from build123d import *

# Parameters (mm, degrees)
F_5_0MM_DOWEL_HOLE1_D                     = 5
F_5_0MM_DOWEL_HOLE1_DEPTH                 = 12
F_5_0MM_DOWEL_HOLE1_CSINK_D               = 5.05
F_5_0MM_DOWEL_HOLE1_CSINK_ANGLE           = 90
F_5_0MM_DOWEL_HOLE1_TIP                   = 1.502151548
F_5_0MM_DOWEL_HOLE1_ON_FACE_2_D           = 5
F_5_0MM_DOWEL_HOLE1_ON_FACE_2_DEPTH       = 12
F_5_0MM_DOWEL_HOLE1_ON_FACE_2_CSINK_D     = 5.05
F_5_0MM_DOWEL_HOLE1_ON_FACE_2_CSINK_ANGLE = 90
F_5_0MM_DOWEL_HOLE1_ON_FACE_2_TIP         = 1.502151548
F_5_0MM_DOWEL_HOLE1_ON_FACE_3_D           = 5
F_5_0MM_DOWEL_HOLE1_ON_FACE_3_DEPTH       = 12
F_5_0MM_DOWEL_HOLE1_ON_FACE_3_CSINK_D     = 5.05
F_5_0MM_DOWEL_HOLE1_ON_FACE_3_CSINK_ANGLE = 90
F_5_0MM_DOWEL_HOLE1_ON_FACE_3_TIP         = 1.502151548
F_5_0MM_DOWEL_HOLE1_ON_FACE_4_D           = 5
F_5_0MM_DOWEL_HOLE1_ON_FACE_4_DEPTH       = 12
F_5_0MM_DOWEL_HOLE1_ON_FACE_4_CSINK_D     = 5.05
F_5_0MM_DOWEL_HOLE1_ON_FACE_4_CSINK_ANGLE = 90
F_5_0MM_DOWEL_HOLE1_ON_FACE_4_TIP         = 1.502151548
M12_TAPPED_HOLE1_D                        = 10.2


with BuildPart() as part:
    # Sketch1 → Revolve1 (revolve)
    with BuildSketch(Plane.XY, mode=Mode.PRIVATE) as revolve1_sk:
        Polygon((0, 6.25), (49, 6.25), (49.5, 5.75), (57, 5.75), (57, -5.75), (0, -5.75), align=None)
    revolve(revolve1_sk.sketch.rotate(Axis((0, 0, 0), (0, 1, 0)), 90), axis=Axis((0, 0, 0), (0, 1, 0)))

    # Ø5.0mm Dowel Hole1
    with Locations(Plane(origin=(57, 0, 0), x_dir=(0, 0, 1), z_dir=(1, 0, 0))):
        with Locations((0, 0)):
            CounterSinkHole(F_5_0MM_DOWEL_HOLE1_D / 2, F_5_0MM_DOWEL_HOLE1_CSINK_D / 2, depth=F_5_0MM_DOWEL_HOLE1_DEPTH, counter_sink_angle=F_5_0MM_DOWEL_HOLE1_CSINK_ANGLE)
            with Locations((0, 0, -(F_5_0MM_DOWEL_HOLE1_DEPTH + F_5_0MM_DOWEL_HOLE1_TIP / 2))):  # 118° drill point
                Cone(0, F_5_0MM_DOWEL_HOLE1_D / 2, F_5_0MM_DOWEL_HOLE1_TIP, mode=Mode.SUBTRACT)

    # Ø5.0mm Dowel Hole1 on face 2
    with Locations(Plane.XY.offset(57)):
        with Locations((0, 0)):
            CounterSinkHole(F_5_0MM_DOWEL_HOLE1_ON_FACE_2_D / 2, F_5_0MM_DOWEL_HOLE1_ON_FACE_2_CSINK_D / 2, depth=F_5_0MM_DOWEL_HOLE1_ON_FACE_2_DEPTH, counter_sink_angle=F_5_0MM_DOWEL_HOLE1_ON_FACE_2_CSINK_ANGLE)
            with Locations((0, 0, -(F_5_0MM_DOWEL_HOLE1_ON_FACE_2_DEPTH + F_5_0MM_DOWEL_HOLE1_ON_FACE_2_TIP / 2))):  # 118° drill point
                Cone(0, F_5_0MM_DOWEL_HOLE1_ON_FACE_2_D / 2, F_5_0MM_DOWEL_HOLE1_ON_FACE_2_TIP, mode=Mode.SUBTRACT)

    # Ø5.0mm Dowel Hole1 on face 3
    with Locations(Plane(origin=(-57, 0, 0), x_dir=(0, 0, -1), z_dir=(-1, 0, 0))):
        with Locations((0, 0)):
            CounterSinkHole(F_5_0MM_DOWEL_HOLE1_ON_FACE_3_D / 2, F_5_0MM_DOWEL_HOLE1_ON_FACE_3_CSINK_D / 2, depth=F_5_0MM_DOWEL_HOLE1_ON_FACE_3_DEPTH, counter_sink_angle=F_5_0MM_DOWEL_HOLE1_ON_FACE_3_CSINK_ANGLE)
            with Locations((0, 0, -(F_5_0MM_DOWEL_HOLE1_ON_FACE_3_DEPTH + F_5_0MM_DOWEL_HOLE1_ON_FACE_3_TIP / 2))):  # 118° drill point
                Cone(0, F_5_0MM_DOWEL_HOLE1_ON_FACE_3_D / 2, F_5_0MM_DOWEL_HOLE1_ON_FACE_3_TIP, mode=Mode.SUBTRACT)

    # Ø5.0mm Dowel Hole1 on face 4
    with Locations(Plane(origin=(0, 0, -57), x_dir=(-1, 0, 0), z_dir=(0, 0, -1))):
        with Locations((0, 0)):
            CounterSinkHole(F_5_0MM_DOWEL_HOLE1_ON_FACE_4_D / 2, F_5_0MM_DOWEL_HOLE1_ON_FACE_4_CSINK_D / 2, depth=F_5_0MM_DOWEL_HOLE1_ON_FACE_4_DEPTH, counter_sink_angle=F_5_0MM_DOWEL_HOLE1_ON_FACE_4_CSINK_ANGLE)
            with Locations((0, 0, -(F_5_0MM_DOWEL_HOLE1_ON_FACE_4_DEPTH + F_5_0MM_DOWEL_HOLE1_ON_FACE_4_TIP / 2))):  # 118° drill point
                Cone(0, F_5_0MM_DOWEL_HOLE1_ON_FACE_4_D / 2, F_5_0MM_DOWEL_HOLE1_ON_FACE_4_TIP, mode=Mode.SUBTRACT)

    # M12 Tapped Hole1 (through all)
    with Locations(Plane(origin=(0, 6.25, 0), x_dir=(1, 0, 0), z_dir=(0, 1, 0))):
        with Locations((0, 0)):
            Hole(M12_TAPPED_HOLE1_D / 2)


solid = part.part
Verification items for the finished model (mm, model axes). A direction names the side the tool comes from. Give positions to 0.01 mm unless a question says otherwise; leave off trailing zeros.
(1) Material ranges on line 1 (Z direction, x = 0, y = -2.75); line 2 (Y direction, x = 54.5, z = 0); line 3 (X direction, y = 3.5, z = 0.5), recorded low to high.
(2) Gauge pin test, flat ends, axial feed: pin 1 (1 mm diameter, centred on x = 6, y = 2, fed in from +Z); pin 2 (6 mm diameter, centred on x = 0, y = 0, fed in from +Z); pin 3 (5 mm diameter, centred on x = 7.5, y = -3.5, fed in from -Z); pin 4 (3 mm diameter, centred on x = 23.5, y = 2.5, fed in from -Z). Record the tip position at first contact, or that the pin passes through.
(3) Access from +Z, -Z, +X, -X, +Y, -Y to the whole of each face (thin tool, end or side, straight path). Record for faces 1 (the face through (0.54, -2.44, 50.9)), 2 (the face through (-0.54, -2.44, -50.9)), 3 (the face through (-50.9, 2.44, -0.54)).
(4) Mould release check, pull along Z, two halves, no side actions. Record for faces 4 (the face through (-0.094, -0.424, 43.759)), 5 (the face through (-47, 5.75, -17)), 6 (the face through (50.9, 2.44, 0.54)): +Z half, -Z half, draft (parallel to the pull), parting line (faces both ways), or undercut.
Worked out:
1. line 1: z = -57 to -5.1, 5.1 to 57
1. line 2: y = -5.75 to -2.5, 2.5 to 5.75
1. line 3: x = -57 to -5.08, 5.08 to 57
2. pin 1: stops at z = 56.73
2. pin 2: stops at z = 57
2. pin 3: stops at z = -56.78
2. pin 4: stops at z = -52.58
3. face 1: +Z
3. face 2: -Z
3. face 3: -X
4. face 4: +Z half
4. face 5: draft
4. face 6: undercut
